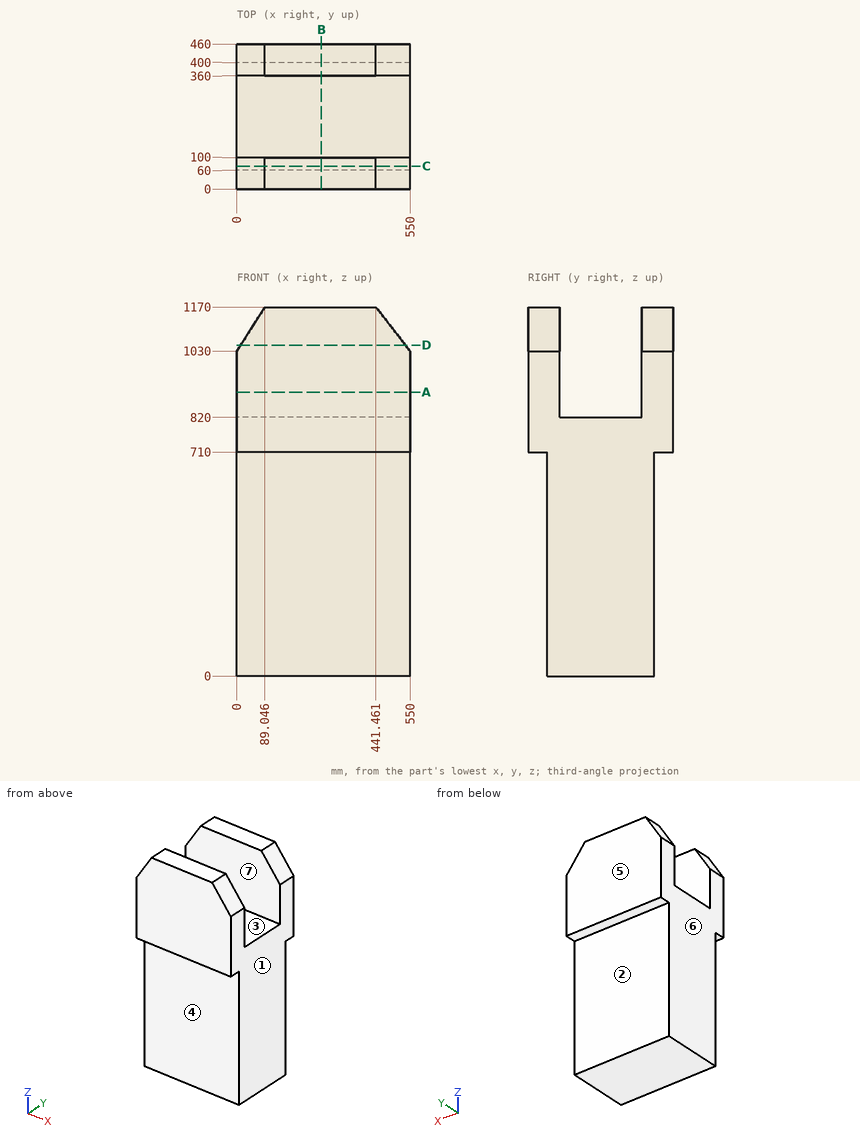
Drawing for the job (mm, zero at the part's lowest x, y, z). A direction names the side the tool comes from. Give positions to 0.01 mm unless a question says otherwise; leave off trailing zeros. Loops run counter-clockwise (first coordinate to the right, second up) from the corner with the lowest first, then second, coordinate; pieces in that order, holes last.
Item 1: Drill centre lines: line 1 along Y through (x, z) = (120.5, 1097.5); line 2 along Y through (x, z) = (195.5, 191); line 3 along Z through (x, y) = (455.5, 190). Where is each one in solid material? Low to high.
Check values:
line 1: y = 0 to 100, 360 to 460
line 2: y = 60 to 400
line 3: z = 0 to 820
Item 2: Which spindle directions (+Z, -Z, +X, -X, +Y, -Y) get a long thin tool onto all of the face, cutting with end or side? Do the marked faces 1, 2, 3 and 4. Say none if no direction does.
Check values:
face 1: +Z, -Z, +X, +Y, -Y
face 2: -Z, +X, -X, +Y
face 3: +Z, +X, -X
face 4: -Z, +X, -X, -Y
Item 3: Drop flat-ended pins along their axis: P1, Ø18, axis at x = 166.5, y = 39.5, coming from the -Z side; P2, Ø4, axis at x = 60, y = 364.5, coming from the +Z side; P3, Ø1, axis at x = 119, z = 191.5, coming from the -Y side. Give the stop position or say it passes through.
Check values:
P1: stops at z = 710
P2: stops at z = 1127.48
P3: stops at y = 60
Item 4: Slice it at A-A (z = 900). Write the cut outline in (x, y), plus the area to 3 significant figures.
Check values:
outline: (0, 0) - (550, 0) - (550, 100) - (0, 100) - close; (0, 360) - (550, 360) - (550, 460) - (0, 460) - close
area: 110,000 mm2
Item 5: Mould opens along Y. For the marked faces 5, 6 and 7 say: +Y half, -Y half, draft (parallel to the pull), parting line (faces both ways), or undercut.
Check values:
face 5: +Y half
face 6: draft
face 7: undercut
Item 6: Slice it at C-C (y = 73). Write the cut outline in (x, z).
Check values:
outline: (0, 0) - (550, 0) - (550, 1030) - (441.46, 1170) - (89.05, 1170) - (0, 1030) - close
Item 7: Slice it at B-B (x = 268.5). Write the cut outline in (y, z), plus the area to 3 significant figures.
Check values:
outline: (0, 710) - (60, 710) - (60, 0) - (400, 0) - (400, 710) - (460, 710) - (460, 1170) - (360, 1170) - (360, 820) - (100, 820) - (100, 1170) - (0, 1170) - close
area: 362,000 mm2
Item 8: Slice it at D-D (z = 1049.5). Write the cut outline in (x, y).
Check values:
outline: (12.4, 0) - (534.88, 0) - (534.88, 100) - (12.4, 100) - close; (12.4, 360) - (534.88, 360) - (534.88, 460) - (12.4, 460) - close
